Could you check a few things on this drawing? It's one solid part, dimensions in mm from its lowest x, y, z. Coordinates: 2 decimals unless noted, no trailing zeros. Write each loop counter-clockwise with the first axis right and the second up, starting at its lowest first coordinate (ties: lowest second). Pieces come first, ordered by that corner, then holes.
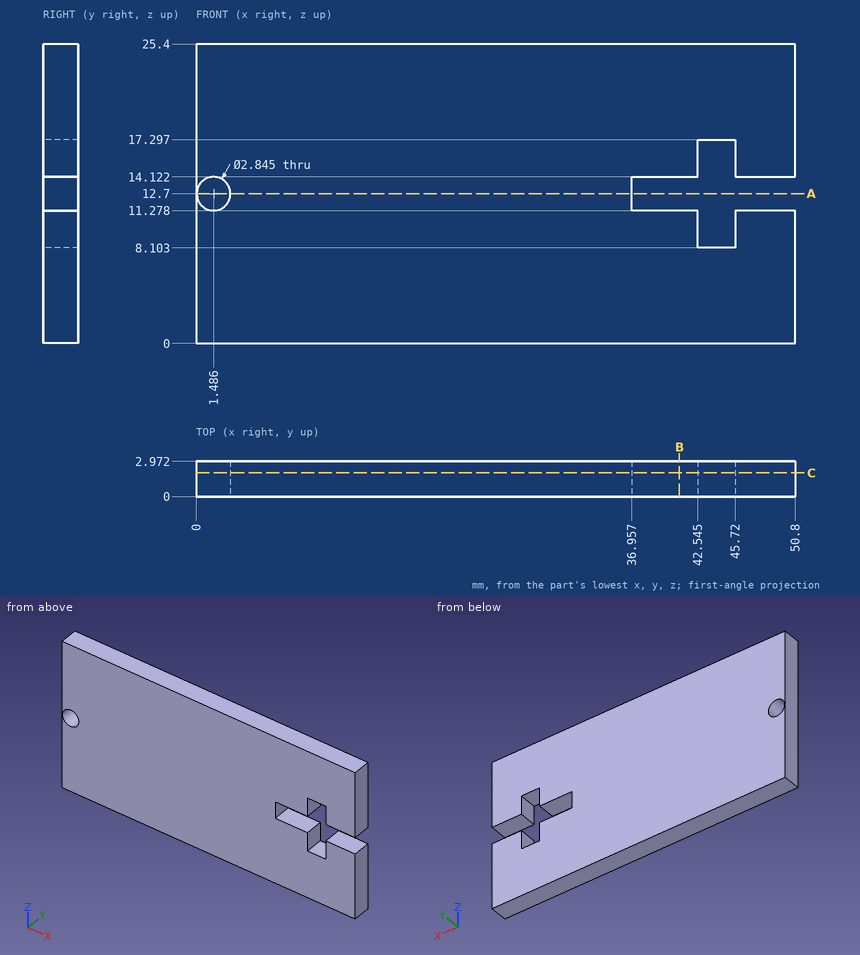
1) Imagine slicing it at C-C on y = 2. Please give me the cut outline in (x, z) (1 decimal).
Values follow:
outline: (0, 0) - (50.8, 0) - (50.8, 11.3) - (45.7, 11.3) - (45.7, 8.1) - (42.5, 8.1) - (42.5, 11.3) - (37, 11.3) - (37, 14.1) - (42.5, 14.1) - (42.5, 17.3) - (45.7, 17.3) - (45.7, 14.1) - (50.8, 14.1) - (50.8, 25.4) - (0, 25.4) - close; hole circle Ø2.8 at (1.5, 12.7)
2) Imagine slicing it at B-B on x = 41. Please give me the cut outline in (y, z).
Values follow:
outline: (0, 0) - (2.97, 0) - (2.97, 11.28) - (0, 11.28) - close; (0, 14.12) - (2.97, 14.12) - (2.97, 25.4) - (0, 25.4) - close
3) Imagine slicing it at A-A on z = 12.7. Please give me the cut outline in (x, y), then the cut area to 3 significant figures.
Values follow:
outline: (0, 0) - (0.06, 0) - (0.06, 2.97) - (0, 2.97) - close; (2.91, 0) - (36.96, 0) - (36.96, 2.97) - (2.91, 2.97) - close
area: 101 mm2
4) I need wall thicknesses on probe 1 along X at (y, z) = (1.6, 8.75) (1 decimal); probe 2 along Z at (x, y) = (44.5, 2.5); probe 3 along X at (y, z) = (1.35, 13.25) (1 decimal). Which ranges of each line are inside material? Lowest first, please.
Values follow:
probe 1: x = 0 to 42.5, 45.7 to 50.8
probe 2: z = 0 to 8.1, 17.3 to 25.4
probe 3: x = 0 to 0.2, 2.8 to 37
5) Will these pins go through, and if not, where does the flat tip stop? pin 1 (1.5 mm diameter, centred on x = 40, y = 1.5, fed in from -Z); pin 2 (1.4 mm diameter, centred on y = 2, z = 13, fed in from +X).
Values follow:
pin 1: stops at z = 0
pin 2: stops at x = 36.96
